Can you work these out from the model? Positions are in its coordinate system, mm. A direction names the side the tool comes from. Give positions to 0.01 mm unless a question says otherwise; leave off trailing zeros. Order: outer loops, then holes, each group sorted by start corner. A loop starts at its lowest first (then second) coordinate and runs counter-clockwise, first axis right, second up. Notation, with made-up numbers: (8, -37.75) -> (65, -37.75) arc R22 cw to (65, -24.75) -> close; hole circle Ø4 at (-4.75, -39.5). An arc over 180 degrees is marked (long way). Answer as CSV lines item,"result".
```python
from build123d import *

# Parameters (mm, degrees)
SKETCH4_R               = 1.7272
CUT_EXTRUDE1_DEPTH      = 5.984800038
CUT_EXTRUDE1_DEPTH_BACK = 14.77519978
SKETCH5_R               = 1.5875
CUT_EXTRUDE2_DEPTH      = 17.775199622
SKETCH6_R               = 3.175
CUT_EXTRUDE3_DEPTH      = 3.175
BOSS_EXTRUDE1_REACH     = 20.76
FILLET1_R               = 3.175
SKETCH8_R               = 2.5527
CUT_EXTRUDE4_DEPTH      = 19.759999818


with BuildPart() as part:
    # Sketch2 → Revolve1 (revolve)
    with BuildSketch(Plane.XY):
        Polygon((-0.015199868, 29.999999944), (-1.815199824, 29.999999944), (-11.775199716, 29.999999944), (-13.77519978, 29.999999944), (-13.77519978, 25.4), (-2.000000064, 25.4), (-2.000000064, 11.499999987), (0.500000016, 11.499999987), (0.500000016, 6.937499968), (1.770899684, 6.937499968), (1.770899684, 7.9375), (1.770899684, 13.93649994), (2.999999842, 13.93649994), (2.999999842, 43.824999885), (4.984800038, 43.824999885), (4.984800038, 44.824999885), (4.984800038, 54.936499982), (4.984800038, 63.5), (-0.015199868, 63.5), align=None)
    revolve(axis=Axis((0, 0, 0), (1, 0, 0)))

    # Sketch4 → Cut-Extrude1 (cut, two sides)
    with BuildSketch(Plane(origin=(0, 0, 0), x_dir=(0, 0, -1), z_dir=(1, 0, 0))) as cut_extrude1_sk:
        with Locations((0, 58.238499982)):
            Circle(SKETCH4_R)
        with Locations((50.436020463, 29.119249991)):
            Circle(SKETCH4_R)
        with Locations((50.436020463, -29.119249991)):
            Circle(SKETCH4_R)
        with Locations((0, -58.238499982)):
            Circle(SKETCH4_R)
        with Locations((-50.436020463, -29.119249991)):
            Circle(SKETCH4_R)
        with Locations((-50.436020463, 29.119249991)):
            Circle(SKETCH4_R)
        with Locations((-14.928978871, 8.61924997)):
            Circle(SKETCH4_R)
        with Locations((0, 17.23849994)):
            Circle(SKETCH4_R)
        with Locations((14.928978871, 8.61924997)):
            Circle(SKETCH4_R)
        with Locations((14.928978871, -8.61924997)):
            Circle(SKETCH4_R)
        with Locations((0, -17.23849994)):
            Circle(SKETCH4_R)
        with Locations((-14.928978871, -8.61924997)):
            Circle(SKETCH4_R)
    extrude(amount=CUT_EXTRUDE1_DEPTH, mode=Mode.SUBTRACT)
    extrude(cut_extrude1_sk.sketch, amount=-CUT_EXTRUDE1_DEPTH_BACK, mode=Mode.SUBTRACT)

    # Sketch5 → Cut-Extrude2 (cut, through all)
    with BuildSketch(Plane(origin=(2.999999842, 0, 0), x_dir=(0, 0, -1), z_dir=(1, 0, 0))):
        with Locations((-18.385, 0)):
            Circle(SKETCH5_R)
        with Locations((18.385, 0)):
            Circle(SKETCH5_R)
    extrude(amount=-CUT_EXTRUDE2_DEPTH, mode=Mode.SUBTRACT)

    # Sketch6 → Cut-Extrude3 (cut)
    with BuildSketch(Plane(origin=(2.999999842, 0, 0), x_dir=(0, 0, -1), z_dir=(1, 0, 0))):
        with Locations((-18.385, 0)):
            Circle(SKETCH6_R)
        with Locations((18.385, 0)):
            Circle(SKETCH6_R)
    extrude(amount=-CUT_EXTRUDE3_DEPTH, mode=Mode.SUBTRACT)

    # Sketch7 → Boss-Extrude1 (add, up to next)
    with BuildSketch(Plane.ZY.offset(13.77519978), mode=Mode.PRIVATE) as boss_extrude1_sk1:
        with BuildLine():
            ThreePointArc((25.213720876, 3.070550371), (17.960512242, 17.960512242), (3.070550371, 25.213720876))
            Line((3.070550371, 25.213720876), (25.213720876, 3.070550371))
        make_face()
    boss_extrude1_tool1 = extrude(boss_extrude1_sk1.sketch, amount=-BOSS_EXTRUDE1_REACH, mode=Mode.PRIVATE) - part.part
    add(boss_extrude1_tool1.solids().sort_by_distance((-13.7752, 15.684318, 15.684318))[0])
    # Sketch7 → Boss-Extrude1 (add, up to next)
    with BuildSketch(Plane.ZY.offset(13.77519978), mode=Mode.PRIVATE) as boss_extrude1_sk2:
        with BuildLine():
            Line((-25.213720876, 3.070550371), (-3.070550371, 25.213720876))
            ThreePointArc((-3.070550371, 25.213720876), (-17.960512242, 17.960512242), (-25.213720876, 3.070550371))
        make_face()
    boss_extrude1_tool2 = extrude(boss_extrude1_sk2.sketch, amount=-BOSS_EXTRUDE1_REACH, mode=Mode.PRIVATE) - part.part
    add(boss_extrude1_tool2.solids().sort_by_distance((-13.7752, 15.684318, -15.684318))[0])
    # Sketch7 → Boss-Extrude1 (add, up to next)
    with BuildSketch(Plane.ZY.offset(13.77519978), mode=Mode.PRIVATE) as boss_extrude1_sk3:
        with BuildLine():
            Line((-3.070550371, -25.213720876), (-25.213720876, -3.070550371))
            ThreePointArc((-25.213720876, -3.070550371), (-17.960512242, -17.960512242), (-3.070550371, -25.213720876))
        make_face()
    boss_extrude1_tool3 = extrude(boss_extrude1_sk3.sketch, amount=-BOSS_EXTRUDE1_REACH, mode=Mode.PRIVATE) - part.part
    add(boss_extrude1_tool3.solids().sort_by_distance((-13.7752, -15.684318, -15.684318))[0])
    # Sketch7 → Boss-Extrude1 (add, up to next)
    with BuildSketch(Plane.ZY.offset(13.77519978), mode=Mode.PRIVATE) as boss_extrude1_sk4:
        with BuildLine():
            ThreePointArc((3.070550371, -25.213720876), (17.960512242, -17.960512242), (25.213720876, -3.070550371))
            Line((25.213720876, -3.070550371), (3.070550371, -25.213720876))
        make_face()
    boss_extrude1_tool4 = extrude(boss_extrude1_sk4.sketch, amount=-BOSS_EXTRUDE1_REACH, mode=Mode.PRIVATE) - part.part
    add(boss_extrude1_tool4.solids().sort_by_distance((-13.7752, -15.684318, 15.684318))[0])

    # Fillet1
    fillet1_edges = [part.edges().sort_by_distance(p)[0] for p in [
        (-7.887599922, 3.070550371, 25.213720876),
        (-7.887599922, 25.213720876, 3.070550371),
        (-7.887599922, 25.213720876, -3.070550371),
        (-7.887599922, 3.070550371, -25.213720876),
        (-7.887599922, -3.070550371, -25.213720876),
        (-7.887599922, -25.213720876, -3.070550371),
        (-7.887599922, -25.213720876, 3.070550371),
        (-7.887599922, -3.070550371, 25.213720876),
    ]]
    fillet(fillet1_edges, radius=FILLET1_R)

    # Sketch8 → Cut-Extrude4 (cut, through all)
    with BuildSketch(Plane.ZY.offset(13.77519978)):
        with Locations((17.67766951, 17.67766951)):
            Circle(SKETCH8_R)
        with Locations((17.67766951, -17.67766951)):
            Circle(SKETCH8_R)
        with Locations((-17.67766951, -17.67766951)):
            Circle(SKETCH8_R)
        with Locations((-17.67766951, 17.67766951)):
            Circle(SKETCH8_R)
    extrude(amount=-CUT_EXTRUDE4_DEPTH, mode=Mode.SUBTRACT)


solid = part.part
```
Item 1: For faces 1 (the flat face through (1.771, 3.3, 6.4)), 2 (the cylindrical face through (-5.505, 16.7, 20.036)), 3 (the cylindrical face through (-7.8, 0, -25.4)), which set-ups out of +Z, -Z, +X, -X, +Y, -Y let a thin tool reach every point of the face, with its end or its side?
Numbers:
face 1,"+X"
face 2,"+X, -X"
face 3,"-X"
Item 2: Imagine slicing it at D-D, the plane z = 40. Please give me the cut outline in (x, y).
Numbers:
outline,"(-0.02, -49.32) -> (4.98, -49.32) -> (4.98, -17.91) -> (3, -17.91) -> (3, 17.91) -> (4.98, 17.91) -> (4.98, 49.32) -> (-0.02, 49.32) -> close"
Item 3: Imagine slicing it at A-A, the plane y = 0. Give the number of separate pieces and of enclosed holes in the cut face, then the cut area to 3 significant figures.
Numbers:
separate pieces,"4"
enclosed holes,"0"
area,"527 mm²"
Item 4: For pin 1 (8 mm diameter, centred on x = -9.5, z = 10.5, fed in from -Y); pin 2 (2 mm diameter, centred on y = -8.62, z = 14.93, fed in from +X); pin 3 (18.5 mm diameter, centred on y = -0.5, z = 4.5, fed in from -X); pin 4 (4.5 mm diameter, centred on y = 58.24, z = 0, fed in from +X), each with a flat end and sliding along its axis, tell me the tip position at first contact or that it passes through.
Numbers:
pin 1,"stops at y = -29.29"
pin 2,"passes through"
pin 3,"stops at x = -2"
pin 4,"stops at x = 4.98"
Item 5: Please list where these lines run through material, in increasing order: line 1 along Z through (x, y) = (2, 2); line 2 along Y through (x, z) = (-8, 1); line 3 along Y through (x, z) = (-12.25, 17.5).
Numbers:
line 1,"z = -63.47 to -20.85, -15.92 to -13.79, 13.79 to 15.92, 20.85 to 63.47"
line 2,"y = -29.98 to -25.38, 25.38 to 29.98"
line 3,"y = -24.37 to -20.22, -15.13 to -10.78, 10.78 to 15.13, 20.22 to 24.37"
Item 6: Imagine slicing it at C-C, the plane x = -6.25. Please give me the cut outline in (y, z) (3 decimals), then the cut area to 3 significant figures.
Numbers:
outline,"circle Ø60 at (0, 0); hole (-25.332, -1.862) arc R3.175 ccw to (-24.41, -3.874) -> (-3.874, -24.41) arc R3.175 ccw to (-1.862, -25.332) arc R25.4 ccw to (1.862, -25.332) arc R3.175 ccw to (3.874, -24.41) -> (24.41, -3.874) arc R3.175 ccw to (25.332, -1.862) arc R25.4 ccw to (25.332, 1.862) arc R3.175 ccw to (24.41, 3.874) -> (3.874, 24.41) arc R3.175 ccw to (1.862, 25.332) arc R25.4 ccw to (-1.862, 25.332) arc R3.175 ccw to (-3.874, 24.41) -> (-24.41, 3.874) arc R3.175 ccw to (-25.332, 1.862) arc R25.4 ccw to start; hole circle Ø5.105 at (-17.678, -17.678); hole circle Ø5.105 at (-17.678, 17.678); hole circle Ø5.105 at (17.678, -17.678); hole circle Ø5.105 at (17.678, 17.678)"
area,"1,180 mm²"
Item 7: We'd pull the mould along Z, two halves only. Please class faces 4 (the cylindrical face through (-7, -24, -18)), 5 (the flat face through (-7.97, -13.998, 14.286)), 6 (the flat face through (-0.015, 27.3, -13.2)): released by +Z, released by -Z, zero draft, split by the parting line, or undercut.
Numbers:
face 4,"split by the parting line"
face 5,"undercut"
face 6,"zero draft"
